Source: CAD feature listing. Evaluate the final solid. Frame: model axes, mm. A direction names the side the tool comes from. Give positions to 0.01 mm unless a question says otherwise; leave off trailing zeros. Loops run counter-clockwise (first coordinate to the right, second up) from the corner with the lowest first, then second, coordinate; pieces in that order, holes last. Notation, with made-up numbers: M -39.75,-17.75 L -22.75,-17.75 A17 cw -22.75,-12.75 Z; hole C -30.5,-6 d5. An arc over 180 degrees is marked long. Put each result on its own line as item: value.
Autodesk Inventor part; units mm, degrees
ref_plane "YZ Plane" through (0, 0, 0) normal (1, 0, 0) x (0, 1, 0)
ref_plane "XZ Plane" through (0, 0, 0) normal (0, 1, 0) x (-1, 0, 0)
ref_plane "XY Plane" through (0, 0, 0) normal (0, 0, 1) x (1, 0, 0)
sketch "Sketch1" plane through (0, 0, 0) normal (0, 0, 1) x (1, 0, 0)
  point P0 (0, 0)
sketch "Sketch2" plane through (0, 0, 0) normal (0, 0, 1) x (1, 0, 0)
  circle A0 centre (0, 0) radius 5
  circle A1 centre (0, 0) radius 10
  circle A2 centre (0, 0) radius 8 construction
  line L0 (0, 0) -> (8, 0) construction
  dimension "d2" = 16
  dimension "d0" = 10
  dimension "d1" = 20
extrude "Extrusion1" add sketch "Sketch2" along normal blind 6
sketch "Sketch3" plane through (0, 0, 6) normal (0, 0, 1) x (1, 0, 0)
  circle A0 centre (0, 0) radius 6.5
  circle A1 centre (0, 0) radius 10
  dimension "d5" = 13
extrude "Extrusion2" cut sketch "Sketch3" against normal blind 3
sketch "Sketch4" plane through (0, 0, 3) normal (0, 0, 1) x (1, 0, 0)
  circle A0 centre (0, 0) radius 8.8
  circle A1 centre (0, 0) radius 10
  dimension "d8" = 17.6
extrude "Extrusion3" cut sketch "Sketch4" against normal blind 1.15
sketch "Sketch5" plane through (0, 0, 3) normal (0, 0, 1) x (1, 0, 0)
  line L0 (0, 0) -> (8, 0) construction
  circle A0 centre (0, 0) radius 8 construction
  line L1 (8, 0) -> (10, 0) construction
  line L2 (7.8487, -1.0896) -> (9.8109, -1.3619)
  line L3 (9.8109, 1.3619) -> (7.8487, 1.0896)
  arc A1 (7.8487, 1.0896) -> (7.8487, -1.0896) centre (8, 0) ccw
  arc A2 (9.8109, -1.3619) -> (9.8109, 1.3619) centre (10, 0) ccw
  line L4 (7.8487, 1.0896) -> (0, 0) construction
  circle A3 centre (0, 0) radius 10 construction
  point P0 (9, 0)
  dimension "d11" = 16
  dimension "d12" = 1.1
extrude "Extrusion4" cut sketch "Sketch5" against normal up to surface (1.15 mm away)
fillet "Fillet1" radius 0.25 2 edges at (8.7164, -1.21, 2.425) (8.7164, 1.21, 2.425)
hole "Hole1" at (8, 0, 3) direction (0, 0, -1) diameter 1.567 end through all
pattern_circular "Circular Pattern1" count 8 over 360 about axis through (0, 0, -10) along (0, 0, 1) of "Extrusion4", "Fillet1", "Hole1"
chamfer "Chamfer1" distance 0.2 angle 45 5 edges at (-5, 0, 6) (-5, 0, 0) (-6.5, 0, 6) (-10, 0, 0) (-10, 0, 1.85)
properties part number "16_029_X430_FREE_HORN_R1" material "Aluminum 6061"
1. Section query C-C (z = 4.1). Output: boundary loops of the cut face in (x, y), plus the area to 3 significant figures.
Found:
outline: C 0,0 d13; hole C 0,0 d10
area: 54.2 mm^2
2. Material intervals for line 1 (Y direction, x = 0, z = 1.35); line 2 (X direction, y = 0.25, z = 3.05); line 3 (Y direction, x = 4.25, z = 1.8), sorted ascending. Write a range as from..to.
Found:
line 1: -10..-8.78, -7.22..-5, 5..7.22, 8.78..10
line 2: -6.5..-4.99, 4.99..6.5
line 3: -8.89..-2.63, 2.63..8.89
3. Section query A-A (y = 0). State how many separate pieces and enclosed holes the cut face has, plus the area to 3 significant figures.
Found:
separate pieces: 4
enclosed holes: 0
area: 25.9 mm^2
4. Contact query for flat-ended pins moving along their axis: P1, Ø1.5, axis at y = -2.5, z = 4.5, coming from the +X side; P2, Ø1.8, axis at x = 5.66, y = 5.66, coming from the +Z side; P3, Ø1.8, axis at x = 0, y = -8, coming from the -Z side. Output: stop coordinate, or through.
Found:
P1: x = 6.26
P2: z = 1.85
P3: z = 0
5. Access query for faces 4 (the cylindrical face through (-6.9, 0, 2.4)), 5 (the cylindrical face through (0, -6.9, 2.4)), 6 (the cylindrical face through (4.864, 4.895, 2.433)). Directions: +Z, -Z, +X, -X, +Y, -Y. A direction counts if a zero-diameter tool reaches every point of the face in a straight line with its end or side. Return the directions, or none.
Found:
face 4: +Z, -X
face 5: +Z, -Y
face 6: +Z
6. Draft query along Y for faces 1 (the cylindrical face through (0, 6.9, 2.4)), 2 (the cylindrical face through (8.12, -3.39, 2.43)), 3 (the cylindrical face through (-8.765, -0.17, 0.912)). Return one class per face: pulls with the +Y half, pulls with the -Y half, needs draft (parallel to the pull), parting line crosses it, or undercut.
Found:
face 1: pulls with the +Y half
face 2: pulls with the -Y half
face 3: undercut
